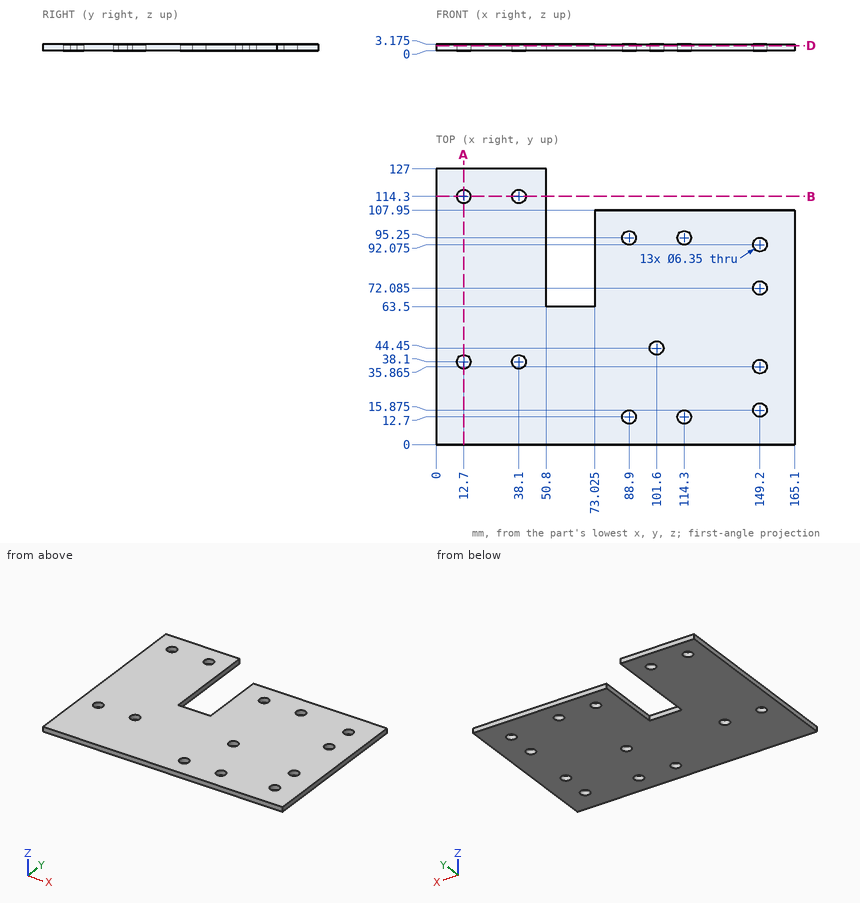
Print and shaded views of the part. All mm, measured from the part's lowest x, y and z. Coordinates: 2 decimals unless noted, no trailing zeros. Write each loop counter-clockwise with the first axis right and the second up, starting at its lowest first coordinate (ties: lowest second). Pieces come first, ordered by that corner, then holes.
(1) Cut at D-D, the plane z = 2.4. Count the separate pieces of the cut face and the enclosed holes in it, and give its area (3 significant figures).
(2) Flat gauge pins, fed straight in: pin 1 (1 mm diameter, centred on x = 138, z = 2, fed in from +Y); pin 2 (1 mm diameter, centred on x = 64.5, z = 1, fed in from +Y). Where does each tip first touch, or does it go through?
(3) Cut at B-B, the plane y = 114.3. List the corners of the cut face in (x, z) (1 decimal).
(4) Drill centre lines: probe 1 along X at (y, z) = (114.3, 0.95) (1 decimal); probe 2 along Y at (x, z) = (13, 2.75); probe 3 along X at (y, z) = (64, 1.95) (1 decimal). Where is each one in solid material? Low to high.
(5) Cut at A-A, the plane x = 12.7. List the corners of the cut face in (y, z) (1 decimal), and give its area (3 significant figures).
Geometry says:
1. separate pieces: 1
1. enclosed holes: 13
1. area: 17,400 mm2
2. pin 1: stops at y = 107.95
2. pin 2: stops at y = 63.5
3. outline: (0, 0) - (9.5, 0) - (9.5, 3.2) - (0, 3.2) - close; (15.9, 0) - (34.9, 0) - (34.9, 3.2) - (15.9, 3.2) - close; (41.3, 0) - (50.8, 0) - (50.8, 3.2) - (41.3, 3.2) - close
4. probe 1: x = 0 to 9.5, 15.9 to 34.9, 41.3 to 50.8
4. probe 2: y = 0 to 34.94, 41.26 to 111.14, 117.46 to 127
4. probe 3: x = 0 to 50.8, 73 to 165.1
5. outline: (0, 0) - (34.9, 0) - (34.9, 3.2) - (0, 3.2) - close; (41.3, 0) - (111.1, 0) - (111.1, 3.2) - (41.3, 3.2) - close; (117.5, 0) - (127, 0) - (127, 3.2) - (117.5, 3.2) - close
5. area: 363 mm2
